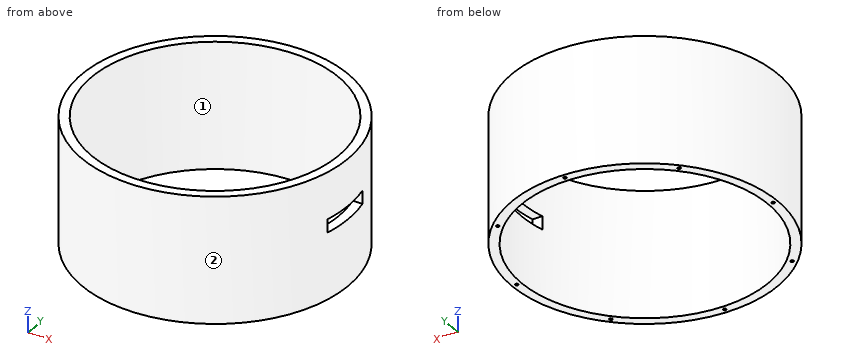
from build123d import *

# Parameters (mm, degrees)
SKETCH1_R                 = 140
SKETCH1_R_2               = 130
BOSS_EXTRUDE1_DEPTH       = 132.6
M4X0_7_TAPPED_HOLE1_D     = 3.3
M4X0_7_TAPPED_HOLE1_DEPTH = 20
M4X0_7_TAPPED_HOLE1_TIP   = 0.991420021
SKETCH5_W                 = 13.9
SKETCH5_H                 = 59.15
CUT_EXTRUDE1_DEPTH        = 140


with BuildPart() as part:
    # Sketch1 → Boss-Extrude1 (new body)
    with BuildSketch(Plane.XY):
        Circle(SKETCH1_R)
        Circle(SKETCH1_R_2, mode=Mode.SUBTRACT)
    extrude(amount=BOSS_EXTRUDE1_DEPTH)

    # M4x0.7 Tapped Hole1
    with Locations(Plane(origin=(0, 0, 0), x_dir=(-1, 0, 0), z_dir=(0, 0, -1))):
        with Locations((0, 135), (135, 0), (95.5, 95.5), (95.5, -95.5), (0, -135), (-95.5, -95.5), (-135, 0), (-95.5, 95.5)):
            Hole(M4X0_7_TAPPED_HOLE1_D / 2, depth=M4X0_7_TAPPED_HOLE1_DEPTH)
            with Locations((0, 0, -(M4X0_7_TAPPED_HOLE1_DEPTH + M4X0_7_TAPPED_HOLE1_TIP / 2))):  # 118° drill point
                Cone(0, M4X0_7_TAPPED_HOLE1_D / 2, M4X0_7_TAPPED_HOLE1_TIP, mode=Mode.SUBTRACT)

    # Sketch5 → Cut-Extrude1 (cut)
    with BuildSketch(Plane(origin=(0, 0, 0), x_dir=(0, 0, -1), z_dir=(1, 0, 0))):
        with Locations((-76.65, 0)):
            Rectangle(SKETCH5_W, SKETCH5_H)
    extrude(amount=CUT_EXTRUDE1_DEPTH, mode=Mode.SUBTRACT)


solid = part.part
Here's how the part is built. I have some questions about the finished solid (model axes, mm). Face numbers are marked on the shaded views. Coordinates: 2 decimals unless noted, no trailing zeros. Order: outer loops, then holes, each group sorted by start corner. A loop starts at its lowest first (then second) coordinate and runs counter-clockwise, first axis right, second up. Notation, with made-up numbers: (84.25, 41.5) - (124.25, 41.5) arc R16 ccw to (124.25, 59.5) - close; hole circle Ø11 at (77, -4.5). An arc over 180 degrees is marked (long way). Use CSV: the item, a comma, the result in double quotes. Start each with the question number.
1. Suppose I cut it at B-B on y = -33. List the corners of the cut face in (x, z) for me, then the cut area to 3 significant figures.
2. Please list where these lines run through material, in increasing order: line 1 (X direction, y = 95.5, z = 11.5); line 2 (X direction, y = 95, z = 10); line 3 (X direction, y = -38.5, z = 12.5). Write a range as from..to.
3. I'm going to push flat-ended pins straight in: pin 1 (10 mm diameter, centred on y = 92, z = 22, fed in from -X); pin 2 (2.5 mm diameter, centred on x = 135, y = 0, fed in from -Z); pin 3 (10 mm diameter, centred on y = 82.5, z = 31, fed in from -X); pin 4 (4 mm diameter, centred on x = 95.5, y = -95.5, fed in from -Z). Where does each tip first touch, or does it pass through?
4. Suppose I cut it at A-A on x = 69. List the corners of the cut face in (y, z) for me, then the cut area to 3 significant figures.
5. If we mould it in two halves opening along Y, with no side actions, what happens to the marked faces 1 and 2? For each: +Y half, -Y half, draft (parallel to the pull), parting line (faces both ways), or undercut.
6. Suppose I cut it at C-C on z = 94.5. List the corners of the cut face in (x, y) for me.
Output:
1,outline,"(-136.06, 0) - (-125.74, 0) - (-125.74, 132.6) - (-136.06, 132.6) - close; (125.74, 0) - (136.06, 0) - (136.06, 132.6) - (125.74, 132.6) - close"
1,area,"2,740 mm2"
2,line 1,"x = -102.37..-97.15, -93.85..-88.2, 88.2..93.85, 97.15..102.37"
2,line 2,"x = -102.83..-97.07, -93.93..-88.74, 88.74..93.93, 97.07..102.83"
2,line 3,"x = -134.6..-124.17, 124.17..134.6"
3,pin 1,"stops at x = -109.69"
3,pin 2,"stops at z = 20.24"
3,pin 3,"stops at x = -116.59"
3,pin 4,"stops at z = 0"
4,outline,"(-121.82, 0) - (-110.18, 0) - (-110.18, 132.6) - (-121.82, 132.6) - close; (110.18, 0) - (121.82, 0) - (121.82, 132.6) - (110.18, 132.6) - close"
4,area,"3,090 mm2"
5,face 1,"undercut"
5,face 2,"parting line"
6,outline,"circle Ø280 at (0, 0); hole circle Ø260 at (0, 0)"
